Autodesk Inventor part; units mm, degrees
ref_plane "YZ Plane" through (0, 0, 0) normal (1, 0, 0) x (0, 1, 0)
ref_plane "XZ Plane" through (0, 0, 0) normal (0, 1, 0) x (-1, 0, 0)
ref_plane "XY Plane" through (0, 0, 0) normal (0, 0, 1) x (1, 0, 0)
sketch "草圖1" plane through (0, 0, 0) normal (0, 1, 0) x (-1, 0, 0)
  circle A0 centre (0, 0) radius 50
  dimension "d0" = 100
extrude "擠出1" add sketch "草圖1" along normal blind 51.6
shell "薄殼1" thickness 3 removed faces 1 at (-9.39, 51.6, -8.8667)
sketch "草圖2" plane through (0, 0, 0) normal (0, -1, 0) x (1, 0, 0)
  circle A0 centre (0, 0) radius 70
  dimension "d4" = 140
extrude "擠出2" add sketch "草圖2" along normal blind 5
sketch "草圖3" plane through (0, 0, 0) normal (0, 1, 0) x (1, 0, 0)
  circle A0 centre (0, 0) radius 60
  line L0 (42.4264, -42.4264) -> (-42.4264, -42.4264)
  line L1 (-42.4264, -42.4264) -> (-42.4264, 42.4264)
  line L2 (-42.4264, 42.4264) -> (42.4264, 42.4264)
  line L3 (42.4264, 42.4264) -> (42.4264, -42.4264)
  line L4 (42.4264, -42.4264) -> (-42.4264, 42.4264) construction
  line L5 (-42.4264, -42.4264) -> (42.4264, 42.4264) construction
  dimension "d7" = 120
hole "孔1" at (-42.4264, 0, 42.4264) at (-42.4264, 0, -42.4264) at (42.4264, 0, -42.4264) at (42.4264, 0, 42.4264) direction (0, -1, 0) diameter 8 depth 8 tip angle 118
sketch "草圖4" plane through (0, 3, 0) normal (0, 1, 0) x (1, 0, 0)
  line L0 (-10, -20) -> (10, -20)
  line L1 (10, -20) -> (10, -10)
  line L2 (10, -10) -> (-10, -10)
  line L3 (-10, -10) -> (-10, -20)
  line L4 (-10, 30) -> (10, 30)
  line L5 (10, 30) -> (10, 40)
  line L6 (10, 40) -> (-10, 40)
  line L7 (-10, 40) -> (-10, 30)
  point P0 (0, 0)
  dimension "d15" = 10
  dimension "d16" = 30
  dimension "d17" = 10
  dimension "d18" = 10
  dimension "d19" = 20
  dimension "d20" = 10
extrude "擠出3" add sketch "草圖4" along normal blind 30
sketch "草圖5" plane through (0, 33, 0) normal (0, 1, 0) x (1, 0, 0)
  line L0 (5, 34.3) -> (-5, 34.3)
  line L1 (-5, 34.3) -> (-5, -14.3)
  line L2 (-5, -14.3) -> (5, -14.3)
  line L3 (5, -14.3) -> (5, 34.3)
  line L4 (5, 34.3) -> (-5, -14.3) construction
  line L5 (-5, 34.3) -> (5, -14.3) construction
  line L6 (10, 30) -> (10, 40)
  line L7 (10, 40) -> (-10, 40)
  line L8 (-10, 30) -> (10, 30)
  line L9 (16.2048, 30) -> (16.2048, -10)
  line L10 (0, 10) -> (16.2048, 10)
  line L11 (10, -10) -> (-10, -10)
  dimension "d23" = 10
  dimension "d24" = 48.6
  dimension "d37" = 5
hole "孔2" at (-5, 33, 14.3) at (5, 33, 14.3) at (5, 33, -34.3) at (-5, 33, -34.3) direction (0, -1, 0) diameter 3 depth 8 tip angle 118
sketch "草圖6" plane through (10, 3, 10) normal (0, 0, -1) x (-1, 0, 0)
  line L0 (20, 0) -> (0, 0)
  line L1 (5, 0) -> (15, 0)
  line L2 (15, 0) -> (15, 20)
  line L3 (15, 20) -> (5, 20)
  line L4 (5, 20) -> (5, 0)
  line L5 (0, 0) -> (0, 30)
  line L6 (20, 0) -> (20, 30)
  point P0 (10, -3)
  dimension "d32" = 5
  dimension "d33" = 5
  dimension "d34" = 20
extrude "擠出4" cut sketch "草圖6" against normal through all
fillet "圓角1" radius 5 2 edges at (5, 23, 15) (-5, 23, 15)
properties part number "底座" material "熱塑性塑膠樹脂"
Model file for the job. Use its own axes, mm. A direction names the side the tool comes from. Coordinates: 2 decimals unless noted, no trailing zeros. Loops run counter-clockwise (first coordinate to the right, second up) from the corner with the lowest first, then second, coordinate; pieces in that order, holes last. Notation, with made-up numbers: (-29, 51.5) -> (28, 51.5) arc R21 cw to (28, 66.5) -> close; hole circle Ø3 at (46.25, 88). An arc over 180 degrees is marked (long way). Answer as a JSON object with one key per item and string values.
Q1. Cut at B-B (z = 3). List the corners of the cut face in (x, y).
Report:
{"outline": "(-69.94, -5) -> (69.94, -5) -> (69.94, 0) -> (49.91, 0) -> (49.91, 51.6) -> (46.9, 51.6) -> (46.9, 3) -> (-46.9, 3) -> (-46.9, 51.6) -> (-49.91, 51.6) -> (-49.91, 0) -> (-69.94, 0) -> close"}
Q2. Pull direction X, two halves, no side cores. Call faces 1 (the flat face through (-48, 0, 17)), 2 (the flat face through (0, 18, -40)), 3 (the cylindrical face through (-55.55, -2.465, 42.594)): released by +X, released by -X, zero draft, split by the parting line, or undercut.
Report:
{"face 1": "zero draft", "face 2": "undercut", "face 3": "split by the parting line"}
Q3. Cut at C-C (x = 36). List the corners of the cut face in (y, z), and give its area (3 significant figures).
Report:
{"outline": "(-5, -60.03) -> (0, -60.03) -> (0, -34.7) -> (51.6, -34.7) -> (51.6, -30.22) -> (3, -30.22) -> (3, 30.22) -> (51.6, 30.22) -> (51.6, 34.7) -> (0, 34.7) -> (0, 60.03) -> (-5, 60.03) -> close", "area": "1,240 mm2"}
Q4. Flat gauge pins, fed straight in: P1, Ø5, axis at y = 8, z = -9.5, coming from the +X side; P2, Ø6, axis at y = 44.5, z = -28, coming from the +X side; P3, Ø8, axis at x = -48, y = 39.5, coming from the +Z side. Where does each tip first touch, or does it go through?
Report:
{"P1": "stops at x = 49.51", "P2": "stops at x = 43.3", "P3": "stops at z = 23.75"}
Q5. 3-axis set-ups, long thin cutter, end or side, ignore diameter. For faces 4 (the flat face through (0, 33, 15)), 5 (the flat face through (5, 11, 15)), 6 (the cylindrical face through (39.05, -2.54, -40.28)): which of +Z, -Z, +X, -X, +Y, -Y reach the whole face in a straight line?
Report:
{"face 4": "+Y", "face 5": "+Z", "face 6": "+Y, -Y"}
Q6. Probe probe 1 along Z at (x, y) = (0, 20); probe 2 along X at (y, z) = (30, -34); probe 3 along Z at (x, y) = (-5, 29). List the from-to ranges inside material, lowest first.
Report:
{"probe 1": "z = -50 to -47, -40 to -30", "probe 2": "x = -36.66 to -32.45, -10 to -6.47, -3.53 to 3.53, 6.47 to 10, 32.45 to 36.66", "probe 3": "z = -49.75 to -46.73, -40 to -35.8, -32.8 to -30, 10 to 12.8, 15.8 to 20, 46.73 to 49.75"}
Q7. Cut at D-D (y = 39). List the corners of the cut face in (x, z).
Report:
{"outline": "circle Ø100 at (0, 0); hole circle Ø94 at (0, 0)"}
Q8. Cut at A-A (y = 28). List the corners of the cut face in (x, z).
Report:
{"outline": "circle Ø100 at (0, 0); (-10, -40) -> (10, -40) -> (10, -30) -> (-10, -30) -> close; (-10, 10) -> (10, 10) -> (10, 20) -> (-10, 20) -> close; hole circle Ø94 at (0, 0); hole circle Ø3 at (-5, -34.3); hole circle Ø3 at (-5, 14.3); hole circle Ø3 at (5, -34.3); hole circle Ø3 at (5, 14.3)"}
